from build123d import *

# Parameters (mm, degrees)
F0_R     = 20.32
F0_R_2   = 4.064
F1_DEPTH = 0.508
F3_DEPTH = 25.4


with BuildPart() as f1:
    # F0 (on Front) → F1 (new body, symmetric)
    with BuildSketch(Plane.XZ):
        Circle(F0_R)
        Circle(F0_R_2, mode=Mode.SUBTRACT)
    extrude(amount=F1_DEPTH, both=True)

    # F2 (on face) → F3 (cut)
    with BuildSketch(Plane.XZ.offset(0.508)):
        with BuildLine():
            Line((18.6211682286, 8.133541283), (13.8818768391, 6.5936521644))
            ThreePointArc((13.8818768391, 6.5936521644), (12.7288391826, 5.6088649724), (12.6098681383, 4.097194525))
            ThreePointArc((12.6098681383, 4.097194525), (13.5946553303, 2.9441568686), (15.1063257776, 2.8251858242))
            Line((15.1063257776, 2.8251858242), (19.8456171671, 4.3650749428))
            ThreePointArc((19.8456171671, 4.3650749428), (19.3254684111, 6.2792253257), (18.6211682286, 8.133541283))
        make_face()
        with BuildLine():
            ThreePointArc((10.284065937, -17.5254211876), (11.9437963266, -16.4392253257), (13.4897148755, -15.1963809039))
            Line((13.4897148755, -15.1963809039), (10.5606717142, -11.1648988524))
            ThreePointArc((10.5606717142, -11.1648988524), (9.2677752071, -10.3726108539), (7.7933271031, -10.726594525))
            ThreePointArc((7.7933271031, -10.726594525), (7.0010391046, -12.0194910321), (7.3550227757, -13.4939391361))
            Line((7.3550227757, -13.4939391361), (10.284065937, -17.5254211876))
        make_face()
        with BuildLine():
            Line((-10.5606717142, -11.1648988524), (-13.4897148755, -15.1963809039))
            ThreePointArc((-13.4897148755, -15.1963809039), (-11.9437963266, -16.4392253257), (-10.284065937, -17.5254211876))
            Line((-10.284065937, -17.5254211876), (-7.3550227757, -13.4939391361))
            ThreePointArc((-7.3550227757, -13.4939391361), (-7.0010391046, -12.0194910321), (-7.7933271031, -10.726594525))
            ThreePointArc((-7.7933271031, -10.726594525), (-9.2677752071, -10.3726108539), (-10.5606717142, -11.1648988524))
        make_face()
        with BuildLine():
            Line((-13.8818768391, 6.5936521644), (-18.6211682286, 8.133541283))
            ThreePointArc((-18.6211682286, 8.133541283), (-19.3254684111, 6.2792253257), (-19.8456171671, 4.3650749428))
            Line((-19.8456171671, 4.3650749428), (-15.1063257776, 2.8251858242))
            ThreePointArc((-15.1063257776, 2.8251858242), (-13.5946553303, 2.9441568686), (-12.6098681383, 4.097194525))
            ThreePointArc((-12.6098681383, 4.097194525), (-12.7288391826, 5.6088649724), (-13.8818768391, 6.5936521644))
        make_face()
    extrude(amount=-F3_DEPTH, mode=Mode.SUBTRACT)


solid = f1.part
Model file for the job. Use its own axes, mm. A direction names the side the tool comes from. Coordinates: 2 decimals unless noted, no trailing zeros. Write each loop counter-clockwise with the first axis right and the second up, starting at its lowest first coordinate (ties: lowest second). Pieces come first, ordered by that corner, then holes. Notation, with made-up numbers: (18, -3) -> (35, -3) arc R25 cw to (35, 24) -> close; hole circle Ø5 at (6, -38.75). An arc over 180 degrees is marked (long way). One line per item, written item: value. Start each with the question number.
1) Pull direction X, two halves, no side cores. Call faces 1 (the face through (0.33, -0.007, 20.317)), 2 (the face through (8.8, -0.01, -15.48)), 3 (the face through (4.23, -0.508, 0.28)): +X half, -X half, draft (parallel to the pull), parting line (faces both ways), or undercut.
2) Slice it at C-C on y = -0.1. Write the cut outline in (x, z), then the cut area to 3 significant figures.
3) Probe probe 1 along Z at (x, y) = (-15, -0.35); probe 2 along Z at (x, y) = (16, 0.1); probe 3 along X at (y, z) = (0.1, 2). List the from-to ranges inside material, lowest first.
4) Slice it at B-B on x = 0. Write the cut outline in (y, z).
5) Slice it at D-D on z = 5. Write the cut outline in (x, y).
6) Flat gauge pin, fed straight in: pin 1 Ø7.5 at (x, z) = (0, 0) entering from +Y. Where does the tip first touch, or does it go through?
7) Slice it at A-A on z = 0. Write the cut outline in (x, y).
8) Which spindle directions (+Z, -Z, +X, -X, +Y, -Y) get a long thin tool onto all of the face, cutting with end or side? Do faces 4 (the face through (-16.218, -0.007, 7.353)), 5 (the face through (16.285, -0.007, 7.374)), 6 (the face through (12.046, -0.007, -13.209)), 7 (the face through (-8.84, -0.01, -15.54)). Say none if no direction does.
Answers follow:
1. face 1: parting line
1. face 2: undercut
1. face 3: draft
2. outline: (-19.85, 4.37) arc R20.32 ccw to (-13.49, -15.2) -> (-10.56, -11.16) arc R1.98 cw to (-7.36, -13.49) -> (-10.28, -17.53) arc R20.32 ccw to (10.28, -17.53) -> (7.36, -13.49) arc R1.98 cw to (10.56, -11.16) -> (13.49, -15.2) arc R20.32 ccw to (19.85, 4.37) -> (15.11, 2.83) arc R1.98 cw to (13.88, 6.59) -> (18.62, 8.13) arc R20.32 ccw to (-18.62, 8.13) -> (-13.88, 6.59) arc R1.98 cw to (-15.11, 2.83) -> close; hole circle Ø8.13 at (0, 0)
2. area: 1,140 mm2
3. probe 1: -13.71 to 2.79, 6.96 to 13.71
3. probe 2: -12.53 to 3.12, 7.28 to 12.53
3. probe 3: -20.22 to -3.54, 3.54 to 20.22
4. outline: (-0.51, -20.32) -> (0.51, -20.32) -> (0.51, -4.06) -> (-0.51, -4.06) -> close; (-0.51, 4.06) -> (0.51, 4.06) -> (0.51, 20.32) -> (-0.51, 20.32) -> close
5. outline: (-12.53, -0.51) -> (12.53, -0.51) -> (12.53, 0.51) -> (-12.53, 0.51) -> close
6. pin 1: through
7. outline: (-20.32, -0.51) -> (-4.06, -0.51) -> (-4.06, 0.51) -> (-20.32, 0.51) -> close; (4.06, -0.51) -> (20.32, -0.51) -> (20.32, 0.51) -> (4.06, 0.51) -> close
8. face 4: -X, +Y, -Y
8. face 5: +X, +Y, -Y
8. face 6: -Z, +Y, -Y
8. face 7: +Y, -Y
